Part model, mm, in its own coordinate system. A direction names the side the tool comes from. Give positions to 0.01 mm unless a question says otherwise; leave off trailing zeros. Order: outer loops, then holes, each group sorted by start corner. A loop starts at its lowest first (then second) coordinate and runs counter-clockwise, first axis right, second up. Notation, with made-up numbers: M 55.5,53.5 L 103.5,53.5 A23 ccw 103.5,64.5 Z; hole C -14.75,-1 d4. An arc over 180 degrees is marked long. One line per question, with ' | ' between items.
```python
from build123d import *

# Parameters (mm, degrees)
F0_W      = 36
F0_H      = 36
F1_DEPTH  = 56
F2_W      = 21
F2_H      = 21
F2_R      = 2.6
F3_DEPTH  = 50
F4_W      = 21
F4_H      = 21
F4_R      = 2.6
F5_DEPTH  = 50
F6_R      = 4.35
F7_DEPTH  = 5.5
F8_R      = 4.35
F9_DEPTH  = 5.5
F10_R     = 4.35
F11_DEPTH = 5.5
F12_R     = 4.35
F13_DEPTH = 5.5


with BuildPart() as f1:
    # F0 (on Top) → F1 (new body)
    with BuildSketch(Plane.XY):
        with Locations((18, 18)):
            Rectangle(F0_W, F0_H)
    extrude(amount=F1_DEPTH)

    # F2 (on face) → F3 (cut)
    with BuildSketch(Plane.XZ):
        with Locations((18, 18)):
            Rectangle(F2_W, F2_H)
        with Locations((18, 38.5)):
            Circle(F2_R)
    extrude(amount=-F3_DEPTH, mode=Mode.SUBTRACT)

    # F4 (on face) → F5 (cut)
    with BuildSketch(Plane.YZ.offset(36)):
        with Locations((18, 38)):
            Rectangle(F4_W, F4_H)
        with Locations((18, 17.5)):
            Circle(F4_R)
    extrude(amount=-F5_DEPTH, mode=Mode.SUBTRACT)

    # F6 (on face) → F7 (cut)
    with BuildSketch(Plane.YZ.offset(36)):
        with Locations((18, 17.5)):
            Circle(F6_R)
    extrude(amount=-F7_DEPTH, mode=Mode.SUBTRACT)

    # F8 (on face) → F9 (cut)
    with BuildSketch(Plane(origin=(0, 0, 0), x_dir=(0, -1, 0), z_dir=(-1, 0, 0))):
        with Locations((-18, 17.5)):
            Circle(F8_R)
    extrude(amount=-F9_DEPTH, mode=Mode.SUBTRACT)

    # F10 (on face) → F11 (cut)
    with BuildSketch(Plane(origin=(0, 36, 0), x_dir=(-1, 0, 0), z_dir=(0, 1, 0))):
        with Locations((-18, 38.5)):
            Circle(F10_R)
    extrude(amount=-F11_DEPTH, mode=Mode.SUBTRACT)

    # F12 (on face) → F13 (cut)
    with BuildSketch(Plane.XZ):
        with Locations((18, 38.5)):
            Circle(F12_R)
    extrude(amount=-F13_DEPTH, mode=Mode.SUBTRACT)


solid = f1.part
```
1. Slice it at D-D on y = 18. Give the cut face in (x, z).
Worked out:
outline: M 0,0 L 36,0 L 36,13.15 L 30.5,13.15 L 30.5,14.9 L 28.5,14.9 L 28.5,7.5 L 7.5,7.5 L 7.5,14.9 L 5.5,14.9 L 5.5,13.15 L 0,13.15 Z; M 0,21.85 L 5.5,21.85 L 5.5,20.1 L 7.5,20.1 L 7.5,27.5 L 0,27.5 Z; M 0,48.5 L 36,48.5 L 36,56 L 0,56 Z; M 28.5,20.1 L 30.5,20.1 L 30.5,21.85 L 36,21.85 L 36,27.5 L 28.5,27.5 Z
2. Tool access for faces 1 (the flat face through (18.1, 30.5, 35.7)), 2 (the flat face through (32, 18, 27.5)), 3 (the flat face through (18, 18, 7.5)), 4 (the flat face through (5.5, 18.1, 14.7)): list every direction of +Z, -Z, +X, -X, +Y, -Y with a clear straight run to the whole face (end or side of a thin tool).
Worked out:
face 1: +Y | face 2: +X, -X | face 3: +Y, -Y | face 4: -X
3. Slice it at B-B on z = 11. Give the cut face in (x, y).
Worked out:
outline: M 0,0 L 7.5,0 L 7.5,36 L 0,36 Z; M 28.5,0 L 36,0 L 36,36 L 28.5,36 Z
4. Slice it at A-A on y = 25. Give the cut face in (x, z), then the cut area to 3 significant figures.
Worked out:
outline: M 0,0 L 36,0 L 36,27.5 L 28.5,27.5 L 28.5,7.5 L 7.5,7.5 L 7.5,27.5 L 0,27.5 Z; M 0,48.5 L 36,48.5 L 36,56 L 0,56 Z | area: 840 mm2
5. Drop flat-ended pins along their axis: pin 1 (4.5 mm diameter, centred on y = 17, z = 18, fed in from +X); pin 2 (7 mm diameter, centred on y = 18, z = 17.5, fed in from -X); pin 3 (7 mm diameter, centred on x = 18, z = 38.5, fed in from -Y); pin 4 (1 mm diameter, centred on y = 19, z = 29, fed in from +X). Give the stop position or say it passes through.
Worked out:
pin 1: stops at x = 30.5 | pin 2: stops at x = 5.5 | pin 3: stops at y = 5.5 | pin 4: passes through
6. Slice it at C-C on x = 18. Give the cut face in (y, z).
Worked out:
outline: M 0,0 L 36,0 L 36,7.5 L 0,7.5 Z; M 0,28.5 L 7.5,28.5 L 7.5,35.9 L 5.5,35.9 L 5.5,34.15 L 0,34.15 Z; M 0,42.85 L 5.5,42.85 L 5.5,41.1 L 7.5,41.1 L 7.5,48.5 L 28.5,48.5 L 28.5,41.1 L 30.5,41.1 L 30.5,42.85 L 36,42.85 L 36,56 L 0,56 Z; M 28.5,28.5 L 36,28.5 L 36,34.15 L 30.5,34.15 L 30.5,35.9 L 28.5,35.9 Z
7. Probe L1, parallel to Z at x = 18, y = 34.65; L2, parallel to Z at x = 1, y = 18; L3, parallel to X at y = 32.5, z = 14. List the from-to ranges inside material, lowest first. Write a range as from..to.
Worked out:
L1: z = 0..7.5, 28.5..34.15, 42.85..56 | L2: z = 0..13.15, 21.85..27.5, 48.5..56 | L3: x = 0..7.5, 28.5..36
8. Mould opens along X. For faces 5 (the flat face through (30.5, 17.9, 14.7)), 6 (the flat face through (17.9, 5.5, 35.7)), 7 (the flat face through (17.7, 36, 33.8)) say: released by +X, released by -X, zero draft, split by the parting line, or undercut.
Worked out:
face 5: released by +X | face 6: undercut | face 7: zero draft
